Read the model definition and answer for the solid it produces. Units are mm, in the model's axes. Face numbers are marked on the shaded views. A direction names the side the tool comes from. Give positions to 0.01 mm unless a question says otherwise; leave off trailing zeros. Write each loop counter-clockwise with the first axis right and the second up, starting at its lowest first coordinate (ties: lowest second). Pieces come first, ordered by that corner, then holes. Notation, with made-up numbers: (-7.5, -30.75) -> (45.5, -30.75) arc R27 ccw to (45.5, 5.25) -> close; hole circle Ø7 at (-8.5, 78.25). An arc over 180 degrees is marked (long way). Put each result on its own line as item: value. Start each with the question number.
Autodesk Fusion 360 part; units mm, degrees
sketch "Sketch2" plane through (0, 0, 0) normal (0, 1, 0) x (1, 0, 0)
  line L0 (0, 0) -> (50, 0)
  line L1 (50, 0) -> (50, -15)
  line L2 (50, -15) -> (0, -15)
  line L3 (0, -15) -> (0, 0)
  dimension "d15" = 50
  dimension "d16" = 15
extrude "Extrude1" add sketch "Sketch2" along normal blind 100
shell "Shell2" thickness 1 removed faces 1 at (33.3333, 33.3333, 15)
sketch "Sketch3" plane through (0, 0, 0) normal (0, -1, 0) x (1, 0, 0)
  line L0 (50, 15) -> (0, 15)
  line L1 (0, 15) -> (0, 0)
  line L2 (0, 0) -> (50, 0)
  line L3 (50, 0) -> (50, 15)
  circle A0 centre (25, 7.5) radius 1.5
  dimension "d20" = 3
  dimension "d21" = 25
  dimension "d22" = 7.5
extrude "Extrude2" cut sketch "Sketch3" against normal blind 100 contours A0
sketch "Sketch4" plane through (50, 0, 0) normal (1, 0, 0) x (0, 1, 0)
  line L0 (0, 15) -> (0, 0)
  line L1 (0, 0) -> (100, 0)
  line L2 (100, 0) -> (100, 15)
  line L3 (100, 15) -> (0, 15)
  circle A0 centre (50, 7.5) radius 1.5
  dimension "d25" = 3
  dimension "d26" = 50
  dimension "d27" = 7.5
extrude "Extrude3" cut sketch "Sketch4" against normal blind 50 contours A0
fillet "Fillet1" radius 1 3 edges at (1, 99, 8) (1, 50, 1) (25, 99, 1)
fillet "Fillet2" radius 1 3 edges at (1, 1, 8.5) (1.2929, 1, 1.2929) (25.5, 1, 1)
fillet "Fillet3" radius 1 5 edges at (49, 99, 8.5) (49, 98.7071, 1.2929) (49, 50, 1) (49, 1.2929, 1.2929) (49, 1, 8.5)
equation "Length = 100 mm"
equation "Width = 50 mm"
equation "Height = 15 mm"
equation "Wall = 1 mm"
equation "LPos = Length / 2"
equation "WPos = Width / 2"
equation "HPos = Height / 2"
equation "Screw = 3 mm"
equation "d15 = Width"
equation "d16 = Height"
equation "d17 = Length"
equation "d19 = Wall"
equation "d20 = Screw"
equation "d21 = WPos"
equation "d22 = HPos"
equation "d25 = Screw"
equation "d26 = LPos"
equation "d27 = HPos"
equation "Internal_fillet = 1 mm"
equation "d32 = Internal_fillet"
equation "d34 = Internal_fillet"
equation "d36 = Internal_fillet"
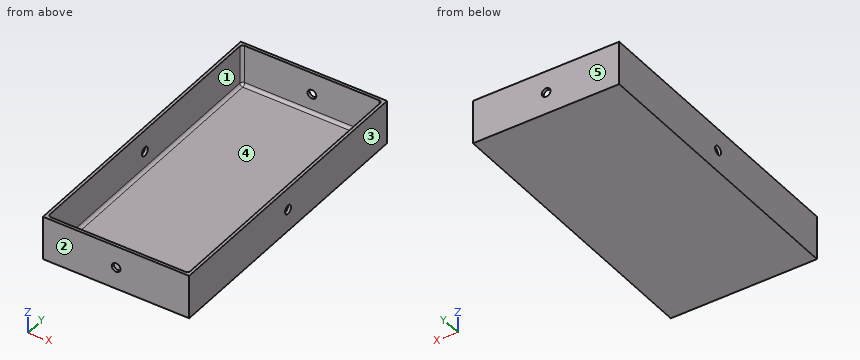
1) Straight lines are drawn through the part: line 1 (Y direction, x = 10, z = 13.5); line 2 (X direction, y = 11.5, z = 8.75); line 3 (Z direction, x = 25, y = 0.75). For each, find the intervals that lie inside material, in ascending order. Write a range as [from, to].
2) Each of these flat-tipped pins is pushed along its axis until it touches: pin 1 Ø10 at (x, y) = (16.5, 20.5) entering from +Z; pin 2 Ø1.8 at (y, z) = (50, 7.5) entering from -X. Where does it stop, or does it pass through?
3) For a pull along Y with two mould halves and no side action, classify the marked faces 1, 2 and 3 as pulls with the +Y half, pulls with the -Y half, needs draft (parallel to the pull), parting line crosses it, or undercut.
4) A cutting plane is placed at A-A on z = 7.5. Give the vertices of the cut face in (x, y).
5) A cutting plane is placed at D-D on z = 13. Give the vertices of the cut face in (x, y), and give its area (3 significant figures).
6) A cutting plane is placed at B-B on x = 25. Give the vertices of the cut face in (y, z), and give its area (3 significant figures).
7) For the marked faces 4 and 5, determine the directions among +Z, -Z, +X, -X, +Y, -Y from which every point of the face is accessible in a straight line to the end or side of a thin tool.
8) A cutting plane is placed at C-C on y = 50. Give the vertices of the cut face in (x, z), and give its area (3 significant figures).
Results found:
1. line 1: y = [0, 1], [99, 100]
1. line 2: x = [0, 1], [49, 50]
1. line 3: z = [0, 6], [9, 15]
2. pin 1: stops at z = 1
2. pin 2: passes through
3. face 1: undercut
3. face 2: pulls with the -Y half
3. face 3: needs draft
4. outline: (0, 0) -> (23.5, 0) -> (23.5, 1) -> (2, 1) arc R1 cw to (1, 2) -> (1, 48.5) -> (0, 48.5) -> close; (0, 51.5) -> (1, 51.5) -> (1, 98) arc R1 cw to (2, 99) -> (23.5, 99) -> (23.5, 100) -> (0, 100) -> close; (26.5, 0) -> (50, 0) -> (50, 48.5) -> (49, 48.5) -> (49, 2) arc R1 cw to (48, 1) -> (26.5, 1) -> close; (26.5, 99) -> (48, 99) arc R1 cw to (49, 98) -> (49, 51.5) -> (50, 51.5) -> (50, 100) -> (26.5, 100) -> close
5. outline: (0, 0) -> (50, 0) -> (50, 100) -> (0, 100) -> close; hole (1, 2) arc R1 ccw to (2, 1) -> (48, 1) arc R1 ccw to (49, 2) -> (49, 98) arc R1 ccw to (48, 99) -> (2, 99) arc R1 ccw to (1, 98) -> close
5. area: 297 mm²
6. outline: (0, 0) -> (100, 0) -> (100, 6) -> (99, 6) -> (99, 2) arc R1 cw to (98, 1) -> (2, 1) arc R1 cw to (1, 2) -> (1, 6) -> (0, 6) -> close; (0, 9) -> (1, 9) -> (1, 15) -> (0, 15) -> close; (99, 9) -> (100, 9) -> (100, 15) -> (99, 15) -> close
6. area: 122 mm²
7. face 4: +Z
7. face 5: +Z, -Z, +X, -X, +Y
8. outline: (0, 0) -> (50, 0) -> (50, 6) -> (49, 6) -> (49, 2) arc R1 cw to (48, 1) -> (2, 1) arc R1 cw to (1, 2) -> (1, 6) -> (0, 6) -> close; (0, 9) -> (1, 9) -> (1, 15) -> (0, 15) -> close; (49, 9) -> (50, 9) -> (50, 15) -> (49, 15) -> close
8. area: 72.4 mm²
